```python
from build123d import *

# Parameters (mm, degrees)
BOSS_EXTRUDE1_DEPTH      = 25.4
BOSS_EXTRUDE1_DEPTH_BACK = 535.94
SKETCH2_R                = 6.35
CUT_EXTRUDE1_DEPTH       = 19


with BuildPart() as part:
    # Sketch1 → Boss-Extrude1 (new, two sides: drawn at the far end of the back side and taken through both)
    with BuildSketch(Plane.XY.offset(1031.10385267).offset(-BOSS_EXTRUDE1_DEPTH_BACK)):
        with BuildLine():
            Line((287.283668248, 598.671970668), (310.642299926, 585.186295534))
            ThreePointArc((310.642299926, 585.186295534), (306.336547982, 564.39371918), (307.203792995, 543.177720091))
            Line((307.203792995, 543.177720091), (268.233668248, 565.676402784))
            Line((268.233668248, 565.676402784), (287.283668248, 598.671970668))
        make_face()
    extrude(amount=BOSS_EXTRUDE1_DEPTH + BOSS_EXTRUDE1_DEPTH_BACK)

    # Sketch2 → Cut-Extrude1 (cut)
    with BuildSketch(Plane(origin=(-43.76981638, 25.270515269, 0), x_dir=(0, 0, 1), z_dir=(-0.8660254037844367, 0.5000000000000036, 0))):
        with Locations(Location((775.671183514, 643.215670872, 0), (0, 0, 270))):
            Circle(SKETCH2_R)
        with Locations(Location((929.595183514, 643.215670872, 0), (0, 0, 270))):
            Circle(SKETCH2_R)
        with Locations(Location((621.747183514, 643.215670872, 0), (0, 0, 270))):
            Circle(SKETCH2_R)
    extrude(amount=-CUT_EXTRUDE1_DEPTH, mode=Mode.SUBTRACT)


solid = part.part
```
For this review, take the finished solid that the model builds, in its own axes (mm). A direction names the side the tool comes from. Coordinates: 2 decimals unless noted, no trailing zeros. Loops run counter-clockwise (first coordinate to the right, second up) from the corner with the lowest first, then second, coordinate; pieces in that order, holes last. Notation, with made-up numbers: (82, 61.25) -> (111, 61.25) arc R14 cw to (111, 83.25) -> close; hole circle Ø5 at (-14.75, 18.25). An arc over 180 degrees is marked (long way). Return JSON: item names as keys, results as strings. Group by question number.
(1) Tool access review of faces 5 (the flat face through (294.34, 572.89, 621.84)), 6 (the flat face through (273.39, 574.61, 771.9)): name each direction out of +Z, -Z, +X, -X, +Y, -Y from which nothing blocks a thin tool from reaching the whole face with its end or side.
(2) Consider section B-B, the plane y = 548. Give the boundary of the cut face in (x, z).
(3) To check wall thickness, follow L1, parallel to Z at x = 287.5, y = 581; L2, parallel to X at y = 578, z = 617; L3, parallel to Y at x = 293.5, z = 625. State the ranges of each line that lie inside material, in increasing order.
(4) For pin 1 Ø5 at (x, z) = (277, 916.5) entering from +Y; pin 2 Ø8 at (x, y) = (289.5, 552) entering from +Z; pin 3 Ø1.5 at (x, z) = (289.5, 868) entering from -Y; pin 4 Ø6 at (x, z) = (273.5, 839) entering from -Y, all flat-tipped, find the tip position at first contact; note any pin that passes through.
(5) Mouldability with a two-part tool opening along X and no side actions: class faces 1 (the flat face through (290, 571, 1056.504)), 2 (the cylindrical face through (286.64, 578.82, 615.55)), 3 (the flat face through (298.799, 592.024, 771.904)), 4 (the flat face through (287.99, 554.27, 771.9)) as pulls with the +X half, pulls with the -X half, needs draft (parallel to the pull), parting line crosses it, or undercut.
(6) Consider section A-A, the plane z = 890. Give the boundary of the cut face in (x, y) (3 decimals), plus the area to 3 significant figures.
Results below:
{
 "1": {"face 5": "none", "face 6": "+Z, -Z, -X, +Y"},
 "2": {"outline": "(298.85, 495.16) -> (306.55, 495.16) -> (306.55, 1056.5) -> (298.85, 1056.5) -> close"},
 "3": {"L1": "z = 495.16 to 616.58, 626.91 to 770.51, 780.84 to 924.43, 934.76 to 1056.5", "L2": "x = 275.35 to 276.87, 293.74 to 308.55", "L3": "y = 551.09 to 571.44, 579.57 to 595.08"},
 "4": {"pin 1": "stops at y = 585.19", "pin 2": "stops at z = 1056.5", "pin 3": "stops at y = 552.97", "pin 4": "stops at y = 560.9"},
 "5": {"face 1": "needs draft", "face 2": "undercut", "face 3": "pulls with the +X half", "face 4": "pulls with the -X half"},
 "6": {"outline": "(268.234, 565.676) -> (307.204, 543.178) arc R86.868 cw to (310.642, 585.186) -> (287.284, 598.672) -> close", "area": "1,300 mm2"}
}
